```python
from build123d import *


with BuildPart() as part:
    # gel → Revolve10 (revolve)
    with BuildSketch(Plane(origin=(0, 0, 0), x_dir=(0, 0, -1), z_dir=(1, 0, 0))):
        with BuildLine():
            Line((45.748610472, 319.342063422), (35.681896581, 309.789108636))
            Line((35.681896581, 309.789108636), (36.026073869, 309.426421451))
            add(Edge.make_bspline(
                [(36.026073869, 309.426421451), (35.418599599, 309.864813343), (34.662663334, 310.791334864), (33.338846471, 311.851350637), (32.195604525, 312.857808267), (31.057999633, 313.930026132), (29.744727596, 314.885066904), (28.443843287, 315.773694322), (27.120617871, 316.745495513), (25.67624262, 317.351925715), (24.437086975, 318.116301123), (23.215591182, 318.685644379), (22.140954977, 319.262698861), (21.068588892, 319.694847458), (19.930975074, 320.193493634), (18.837916971, 320.641634287), (17.733867065, 321.01494492), (16.810008216, 321.249118962), (15.911496119, 321.566233217), (14.864343001, 321.911666773), (13.637151846, 322.313021034), (12.181632664, 322.557718535), (10.750690756, 322.85377071), (9.272215479, 323.156322342), (7.693496909, 323.429691693), (5.699030772, 323.815957427), (4.197169533, 323.839631011), (3.296807109, 324.000001326)],
                knots=[0, 0, 0, 0, 0.060955497, 0.097023752, 0.138612849, 0.185723979, 0.224847013, 0.271346916, 0.31492086, 0.358660312, 0.398942406, 0.433935796, 0.468925884, 0.498724619, 0.528515026, 0.570655164, 0.595402325, 0.623879931, 0.648625043, 0.673368363, 0.714214895, 0.754112569, 0.794010196, 0.833908612, 0.877650512, 0.925245481, 1, 1, 1, 1], degree=3))
            Line((3.296807109, 324.000001326), (0, 324))
            Line((0, 324), (0, 332))
            ThreePointArc((0, 332), (24.81742663, 331.071133347), (49.495985309, 328.289730936))
            Line((49.495985309, 328.289730936), (48.021369991, 318.979376237))
            Line((48.021369991, 318.979376237), (46.09278776, 318.979376237))
            Line((46.09278776, 318.979376237), (45.748610472, 319.342063422))
        make_face()
    revolve(axis=Axis((0, 0, 0), (0, 1, 0)))


solid = part.part
```
CAD build for the part. Positions are in the model's coordinates, mm. Give positions to 0.01 mm unless a question says otherwise; leave off trailing zeros. Order: outer loops, then holes, each group sorted by start corner. A loop starts at its lowest first (then second) coordinate and runs counter-clockwise, first axis right, second up. Notation, with made-up numbers: M 39,51 L 52,51 A23 ccw 52,60 Z; hole C 81,64 d11. An arc over 180 degrees is marked long. Put each result on its own line as item: value. Start each with the question number.
(1) Saw through at A-A, the plane y = 326.5. Write the cut outline in (x, z), then the cut area to 3 significant figures.
(2) Flat gauge pins, fed straight in: pin 1 Ø1 at (x, z) = (-31, -32.5) entering from -Y; pin 2 Ø5 at (x, z) = (32.5, -1) entering from -Y; pin 3 Ø3 at (y, z) = (316.5, -2) entering from +X; pin 4 Ø12 at (x, z) = (35, -20) entering from -Y. Where does each tip first touch, or does it go through?
(3) Mould opens along X. For faces 1 (the conical face through (-14.45, 319.43, -45.87)), 2 (the flat face through (-43, 318.979, 18)), 3 (the conical face through (0, 324, 0)) say: +X half, -X half, draft (parallel to the pull), parting line (faces both ways), or undercut.
(4) Drill centre lines: line 1 along X through (y, z) = (310.75, -28.5); line 2 along X through (y, z) = (310.75, 2.5); line 3 along Y through (x, z) = (34, 1.5). Where is each one in solid material? Low to high.
Check result:
1. outline: C 0,0 d98.43
1. area: 7,610 mm2
2. pin 1: stops at y = 318.08
2. pin 2: stops at y = 310.34
2. pin 3: stops at x = 44.29
2. pin 4: stops at y = 309.43
3. face 1: parting line
3. face 2: draft
3. face 3: undercut
4. line 1: x = -23.11 to -19.64, 19.64 to 23.11
4. line 2: x = -36.61 to -34.52, 34.52 to 36.61
4. line 3: y = 311.29 to 330.25
